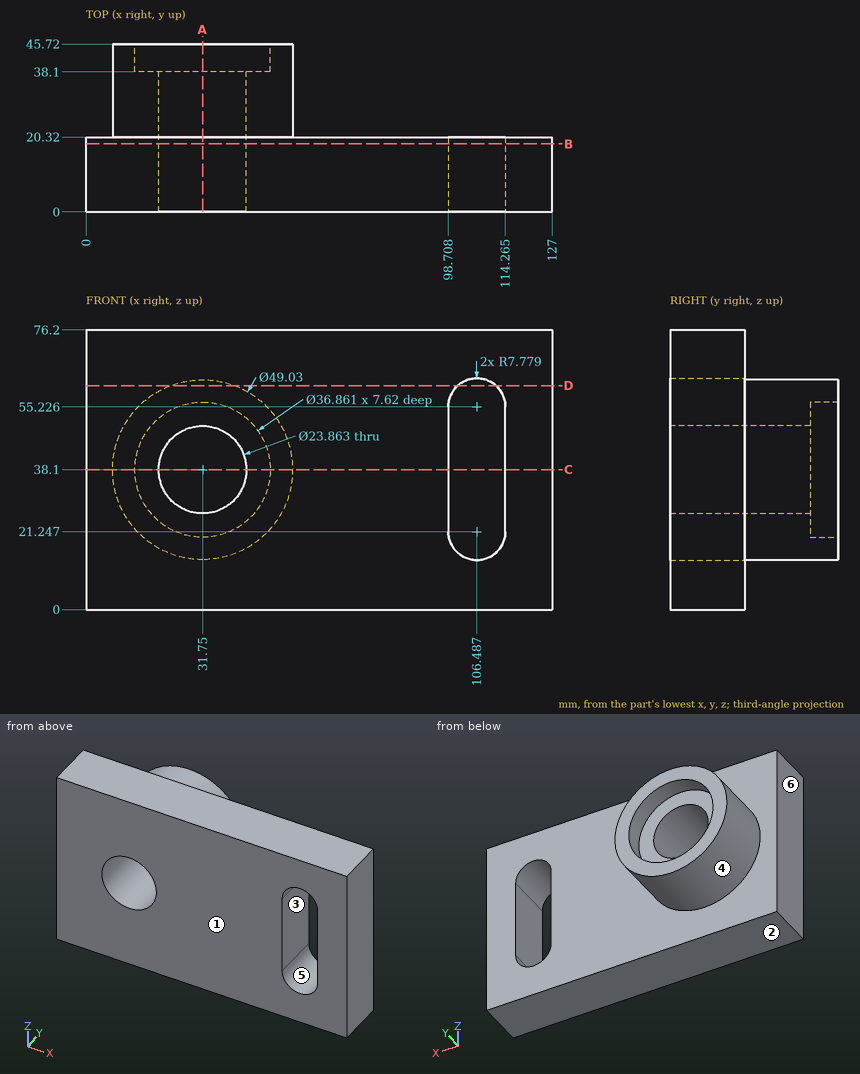
Answer from the drawing. Dimensions are ordinates in mm from the lowest x, y and z of the part. A direction names the side the tool comes from. Round coordinates to 2 decimals unless told otherwise and drop trailing zeros. Order: outer loops, then holes, each group sorted by start corner. A loop starts at its lowest first (then second) coordinate and runs counter-clockwise, first axis right, second up. Notation, with made-up numbers: (-16, 22.25) -> (6, 22.25) arc R25 ccw to (6, 41.25) -> close; hole circle Ø8 at (40, 53.5). An arc over 180 degrees is marked (long way). Answer as CSV lines item,"result".
Q1. A cutting plane is placed at C-C on z = 38.1. Determine the outline of the cut face in (x, y) (1 decimal), plus the area to 3 significant figures.
Computed values:
outline,"(0, 0) -> (19.8, 0) -> (19.8, 38.1) -> (13.3, 38.1) -> (13.3, 45.7) -> (7.2, 45.7) -> (7.2, 20.3) -> (0, 20.3) -> close; (43.7, 0) -> (98.7, 0) -> (98.7, 20.3) -> (56.3, 20.3) -> (56.3, 45.7) -> (50.2, 45.7) -> (50.2, 38.1) -> (43.7, 38.1) -> close; (114.3, 0) -> (127, 0) -> (127, 20.3) -> (114.3, 20.3) -> close"
area,"2,320 mm^2"
Q2. For a pull along Z with two mould halves and no side action, classify the marked faces 1, 2 and 3 as +Z half, -Z half, draft (parallel to the pull), parting line (faces both ways), or undercut.
Computed values:
face 1,"draft"
face 2,"-Z half"
face 3,"undercut"
Q3. Which of the six approach directions +Z, -Z, +X, -X, +Y, -Y give full straight-line access (tool end or side, diameter ignored) to the marked faces 4, 5 and 6?
Computed values:
face 4,"+Y"
face 5,"+Y, -Y"
face 6,"+Z, -Z, -X, +Y, -Y"
Q4. Consider line 1 (X direction, y = 44, z = 38.1) (1 decimal); line 2 (X direction, y = 15, z = 47) (1 decimal); line 3 (Y direction, x = 111, z = 5.5). Determine where each line is inside the solid, lowest interval first. Write a range as from..to.
Computed values:
line 1,"x = 7.2..13.3, 50.2..56.3"
line 2,"x = 0..23.8, 39.7..98.7, 114.3..127"
line 3,"y = 0..20.32"
Q5. A cutting plane is placed at D-D on z = 61. Determine the outline of the cut face in (x, y) (1 decimal), plus the area to 3 significant figures.
Computed values:
outline,"(0, 0) -> (101.3, 0) -> (101.3, 20.3) -> (40.5, 20.3) -> (40.5, 45.7) -> (23, 45.7) -> (23, 20.3) -> (0, 20.3) -> close; (111.7, 0) -> (127, 0) -> (127, 20.3) -> (111.7, 20.3) -> close"
area,"2,810 mm^2"
Q6. A cutting plane is placed at A-A on x = 31.75. Determine the outline of the cut face in (y, z) (1 decimal).
Computed values:
outline,"(0, 0) -> (20.3, 0) -> (20.3, 13.6) -> (45.7, 13.6) -> (45.7, 19.7) -> (38.1, 19.7) -> (38.1, 26.2) -> (0, 26.2) -> close; (0, 50) -> (38.1, 50) -> (38.1, 56.5) -> (45.7, 56.5) -> (45.7, 62.6) -> (20.3, 62.6) -> (20.3, 76.2) -> (0, 76.2) -> close"
Q7. Given pin 1 (8 mm diameter, centred on y = 16.5, z = 43.5, fed in from -X); pin 2 (1.5 mm diameter, centred on x = 41, y = 29.5, fed in from +Z) (1 decimal); pin 3 (18.5 mm diameter, centred on x = 24, z = 39.5, fed in from +Y); pin 4 (23 mm diameter, centred on x = 70.5, z = 20, fed in from +Y), each flat-ended and moving along its own axis, determine where each tip first touches the part or whether it passes through.
Computed values:
pin 1,"stops at x = 0"
pin 2,"stops at z = 61.1"
pin 3,"stops at y = 38.1"
pin 4,"stops at y = 20.32"
Q8. A cutting plane is placed at B-B on y = 18.5. Give the number of separate pieces and of enclosed holes in the cut face, plus the area to 3 significant figures.
Computed values:
separate pieces,"1"
enclosed holes,"2"
area,"8,510 mm^2"
